```python
from build123d import *

# Parameters (mm, degrees)
SKETCH1_R           = 4
SKETCH1_R_2         = 2.5
BOSS_EXTRUDE1_DEPTH = 10
FILLET1_R           = 0.25


with BuildPart() as part:
    # Sketch1 → Boss-Extrude1 (new body)
    with BuildSketch(Plane.XY):
        Circle(SKETCH1_R)
        Circle(SKETCH1_R_2, mode=Mode.SUBTRACT)
    extrude(amount=BOSS_EXTRUDE1_DEPTH)

    # Fillet1
    fillet1_edges = [part.edges().sort_by_distance(p)[0] for p in [
        (-4, 0, 10),
        (-4, 0, 0),
        (-2.5, 0, 0),
        (-2.5, 0, 10),
    ]]
    fillet(fillet1_edges, radius=FILLET1_R)


solid = part.part
```
Could you check a few things on this model? Use its own coordinates, in mm. Give positions to 0.01 mm unless a question says otherwise; leave off trailing zeros. Write each loop counter-clockwise with the first axis right and the second up, starting at its lowest first coordinate (ties: lowest second). Pieces come first, ordered by that corner, then holes. Notation, with made-up numbers: (4.5, 37) - (27.5, 37) arc R17 ccw to (27.5, 59) - close; hole circle Ø7 at (89, -16). An arc over 180 degrees is marked (long way). One line per item, written item: value. Start each with the question number.
Item 1: Please list where these lines run through material, in increasing order: line 1 (Y direction, x = 0, z = 6.25); line 2 (X direction, y = -1.5, z = 2.5); line 3 (Y direction, x = -1.25, z = 8). Write a range as from..to.
Item 2: Imagine slicing it at C-C, the plane z = 7.5. List the corners of the cut face in (x, y) for me.
Item 3: Imagine slicing it at A-A, the plane y = 0. List the corners of the cut face in (x, z) for me.
Item 4: I'm going to push flat-ended pins straight in: pin 1 (1 mm diameter, centred on y = -2.5, z = 2, fed in from -X); pin 2 (2 mm diameter, centred on y = 3, z = 7, fed in from +X); pin 3 (4 mm diameter, centred on y = 2.5, z = 1, fed in from -X). Where does each tip first touch, or does it pass through?
Item 5: If we mould it in two halves opening along X, with no side actions, what happens to faces 1 (the face through (-0.867, -3.905, 4.934)), 2 (the face through (-0.54, -2.44, 4.93)), 3 (the face through (-1, 3, 0))? For each: +X half, -X half, draft (parallel to the pull), parting line (faces both ways), or undercut.
Geometry says:
1. line 1: -4..-2.5, 2.5..4
1. line 2: -3.71..-2, 2..3.71
1. line 3: -3.8..-2.17, 2.17..3.8
2. outline: circle Ø8 at (0, 0); hole circle Ø5 at (0, 0)
3. outline: (-4, 0.25) arc R0.25 ccw to (-3.75, 0) - (-2.75, 0) arc R0.25 ccw to (-2.5, 0.25) - (-2.5, 9.75) arc R0.25 ccw to (-2.75, 10) - (-3.75, 10) arc R0.25 ccw to (-4, 9.75) - close; (2.5, 0.25) arc R0.25 ccw to (2.75, 0) - (3.75, 0) arc R0.25 ccw to (4, 0.25) - (4, 9.75) arc R0.25 ccw to (3.75, 10) - (2.75, 10) arc R0.25 ccw to (2.5, 9.75) - close
4. pin 1: x = -3.46
4. pin 2: x = 3.46
4. pin 3: x = -3.97
5. face 1: parting line
5. face 2: undercut
5. face 3: draft
